The listing builds one solid part. Answer for the finished solid, in the listing's coordinates (mm). Face numbers are marked on the shaded views. A direction names the side the tool comes from. Round coordinates to 2 decimals unless told otherwise and drop trailing zeros. Loops run counter-clockwise (first coordinate to the right, second up) from the corner with the lowest first, then second, coordinate; pieces in that order, holes last. Notation, with made-up numbers: (58, -30.75) -> (112, -30.75) arc R18 cw to (112, -20.75) -> close; hole circle Ø4 at (-22.5, 44.25). An arc over 180 degrees is marked (long way). Write each question's results on one line, items separated by ' | '. Start each with the question number.
(1) For the marked faces 1, 2, 3 and 4, determine the directions among +Z, -Z, +X, -X, +Y, -Y from which every point of the face is accessible in a straight line to the end or side of a thin tool.
(2) The part is cut by section C-C (z = 8.25). Determine the outline of the cut face in (x, y).
(3) Determine the mould class of the marked faces 5, 6, 7 and 8 for opening direction Z: released by +Z, released by -Z, zero draft, split by the parting line, or undercut.
(4) Straight lines are drawn through the part: probe 1 along Y at (x, z) = (-8.55, 0) (3 decimals); probe 2 along Z at (x, y) = (-6.5, -20); probe 3 along X at (y, z) = (-15, 0.75). For each, find the intervals that lie inside material, in ascending order.
(5) The part is cut by section A-A (y = -15). Count the separate pieces of the cut face and the enclosed holes in it, plus the area to 3 significant figures.
(6) The part is cut by section D-D (y = -8). Determine the outline of the cut face in (x, z).
(7) Flat-ended cylindrical pins translate along their axes: pin 1 (7 mm diameter, centred on x = -14.5, y = -18, fed in from +Z); pin 2 (4 mm diameter, centred on y = -5, z = 14.5, fed in from +X). Find the tip coordinate at first contact, or state that the pin passes through.
(8) The part is cut by section B-B (x = -7.5). Determine the outline of the cut face in (y, z) (3 decimals), plus the area to 3 significant figures.
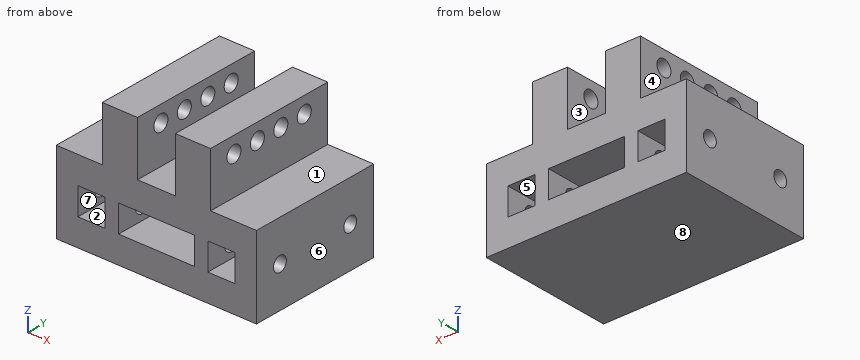
```python
from build123d import *

# Parameters (mm, degrees)
F0_W     = 5
F0_H     = 5
F0_W_2   = 14
F0_W_3   = 6.5
F0_H_2   = 10
F1_DEPTH = 25
F2_R     = 1.5
F3_DEPTH = 37


with BuildPart() as f1:
    # F0 (on Front) → F1 (new body)
    with BuildSketch(Plane.XZ):
        Polygon((-18.5, -7.5), (18.5, -7.5), (18.5, 7.5), (10, 7.5), (3.5, 7.5), (-3.5, 7.5), (-10, 7.5), (-18.5, 7.5), align=None)
        with Locations((-12, 0)):
            Rectangle(F0_W, F0_H, mode=Mode.SUBTRACT)
        Rectangle(F0_W_2, F0_H, mode=Mode.SUBTRACT)
        with Locations((12, 0)):
            Rectangle(F0_W, F0_H, mode=Mode.SUBTRACT)
        with Locations((6.75, 12.5)):
            Rectangle(F0_W_3, F0_H_2)
        with Locations((-6.75, 12.5)):
            Rectangle(F0_W_3, F0_H_2)
    extrude(amount=F1_DEPTH)

    # F2 (on face) → F3 (cut, through all)
    with BuildSketch(Plane(origin=(-18.5, 0, 0), x_dir=(0, -1, 0), z_dir=(-1, 0, 0))):
        with Locations((5, 14.5)):
            Circle(F2_R)
        with Locations((10, 14.5)):
            Circle(F2_R)
        with Locations((15, 14.5)):
            Circle(F2_R)
        with Locations((20, 14.5)):
            Circle(F2_R)
        with BuildLine():
            Line((18.625, 0), (21.375, 0))
            ThreePointArc((21.375, 0), (20, 1.375), (18.625, 0))
        make_face()
        with BuildLine():
            Line((3.625, 0), (6.375, 0))
            ThreePointArc((6.375, 0), (5, 1.375), (3.625, 0))
        make_face()
        with BuildLine():
            ThreePointArc((3.625, 0), (5, -1.375), (6.375, 0))
            Line((6.375, 0), (3.625, 0))
        make_face()
        with BuildLine():
            ThreePointArc((18.625, 0), (20, -1.375), (21.375, 0))
            Line((21.375, 0), (18.625, 0))
        make_face()
    extrude(amount=-F3_DEPTH, mode=Mode.SUBTRACT)


solid = f1.part
```
Checked values:
1) face 1: +Z, +X, +Y, -Y | face 2: +Y, -Y | face 3: +Z, +Y, -Y | face 4: +Z, -X, +Y, -Y
2) outline: (-10, -25) -> (-3.5, -25) -> (-3.5, 0) -> (-10, 0) -> close; (3.5, -25) -> (10, -25) -> (10, 0) -> (3.5, 0) -> close
3) face 5: undercut | face 6: zero draft | face 7: undercut | face 8: released by -Z
4) probe 1: y = -25 to -21.375, -18.625 to -6.375, -3.625 to 0 | probe 2: z = -7.5 to -2.5, 2.5 to 13, 16 to 17.5 | probe 3: x = -18.5 to -14.5, -9.5 to -7, 7 to 9.5, 14.5 to 18.5
5) separate pieces: 3 | enclosed holes: 3 | area: 526 mm2
6) outline: (-18.5, -7.5) -> (18.5, -7.5) -> (18.5, 7.5) -> (10, 7.5) -> (10, 17.5) -> (3.5, 17.5) -> (3.5, 7.5) -> (-3.5, 7.5) -> (-3.5, 17.5) -> (-10, 17.5) -> (-10, 7.5) -> (-18.5, 7.5) -> close; hole (-14.5, -2.5) -> (-9.5, -2.5) -> (-9.5, 2.5) -> (-14.5, 2.5) -> close; hole (-7, -2.5) -> (7, -2.5) -> (7, 2.5) -> (-7, 2.5) -> close; hole (9.5, -2.5) -> (14.5, -2.5) -> (14.5, 2.5) -> (9.5, 2.5) -> close
7) pin 1: stops at z = 7.5 | pin 2: stops at x = 10
8) outline: (-25, -7.5) -> (0, -7.5) -> (0, 17.5) -> (-25, 17.5) -> close; hole circle Ø3 at (-20, 14.5); hole circle Ø2.75 at (-20, 0); hole circle Ø3 at (-15, 14.5); hole circle Ø3 at (-10, 14.5); hole circle Ø3 at (-5, 14.5); hole circle Ø2.75 at (-5, 0) | area: 585 mm2
